```python
from build123d import *

# Parameters (mm, degrees)
F0_W      = 128
F0_H      = 175
F1_DEPTH  = 25
F2_T      = -2.5
F3_R      = 4
F3_R_2    = 1.5
F4_DEPTH  = 20
F7_DEPTH  = 25
F8_R      = 2
F9_DEPTH  = 25
F11_W     = 40
F11_H     = 74
F11_W_2   = 80
F11_H_2   = 15.985015
F12_DEPTH = 36
F13_R     = 1
F15_W     = 5.084744
F15_H     = 25.423729
F16_DEPTH = 47.5


with BuildPart() as f1:
    # F0 (on Front) → F1 (new body)
    with BuildSketch(Plane.XZ):
        Rectangle(F0_W, F0_H)
    extrude(amount=F1_DEPTH)

    # F2
    f2_openings = [f1.faces().sort_by_distance(p)[0] for p in [
        (0, -25, 0),
    ]]
    offset(amount=F2_T, openings=f2_openings)

    # F3 (on Front) → F4 (join)
    with BuildSketch(Plane.XZ):
        with Locations((-37, 47)):
            Circle(F3_R)
        with Locations((-37, 47)):
            Circle(F3_R_2, mode=Mode.SUBTRACT)
        with Locations((37, 47)):
            Circle(F3_R)
        with Locations((37, 47)):
            Circle(F3_R_2, mode=Mode.SUBTRACT)
        with Locations((37, -47)):
            Circle(F3_R)
        with Locations((37, -47)):
            Circle(F3_R_2, mode=Mode.SUBTRACT)
        with Locations((-37, -47)):
            Circle(F3_R)
        with Locations((-37, -47)):
            Circle(F3_R_2, mode=Mode.SUBTRACT)
    extrude(amount=F4_DEPTH)

    # F6 (on Front) → F7 (join)
    with BuildSketch(Plane.XZ):
        with BuildLine():
            Line((-61.93007, -75.520713), (-61.93007, -85.520713))
            Line((-61.93007, -85.520713), (-51.93007, -85.520713))
            ThreePointArc((-51.93007, -85.520713), (-54.690152, -78.280795), (-61.93007, -75.520713))
        make_face()
        with BuildLine():
            ThreePointArc((61.93007, -75.520713), (54.690152, -78.280795), (51.93007, -85.520713))
            Line((51.93007, -85.520713), (61.93007, -85.520713))
            Line((61.93007, -85.520713), (61.93007, -75.520713))
        make_face()
        with BuildLine():
            ThreePointArc((-61.6409, 75.150812), (-54.400982, 77.910894), (-51.6409, 85.150812))
            Line((-51.6409, 85.150812), (-61.6409, 85.150812))
            Line((-61.6409, 85.150812), (-61.6409, 75.150812))
        make_face()
        with BuildLine():
            Line((61.6409, 75.150812), (61.6409, 85.150812))
            Line((61.6409, 85.150812), (51.6409, 85.150812))
            ThreePointArc((51.6409, 85.150812), (54.400982, 77.910894), (61.6409, 75.150812))
        make_face()
    extrude(amount=F7_DEPTH)

    # F8 (on Front) → F9 (cut)
    with BuildSketch(Plane.XZ):
        with Locations((-58.5, 82)):
            Circle(F8_R)
        with Locations((-58.5, -82)):
            Circle(F8_R)
        with Locations((58.5, -82)):
            Circle(F8_R)
        with Locations((58.5, 82)):
            Circle(F8_R)
    extrude(amount=F9_DEPTH, mode=Mode.SUBTRACT)

    # F11 (on offset) → F12 (cut)
    with BuildSketch(Plane.XZ.offset(-10)):
        with Locations((-50, 0)):
            Rectangle(F11_W, F11_H)
        with Locations((50, 0)):
            Rectangle(F11_W, F11_H)
        with Locations((0, 67.007492)):
            Rectangle(F11_W_2, F11_H_2)
        with Locations((0, -67.007492)):
            Rectangle(F11_W_2, F11_H_2)
    extrude(amount=F12_DEPTH, mode=Mode.SUBTRACT)

    # F13
    f13_edges = [f1.edges().sort_by_distance(p)[0] for p in [
        (64, -12.5, 87.5),
        (0, 0, 87.5),
        (64, 0, 62.25),
        (64, 0, -62.25),
        (0, 0, -87.5),
        (-64, 0, 62.25),
        (-64, 0, -62.25),
        (-64, -12.5, 87.5),
    ]]
    fillet(f13_edges, radius=F13_R)

    # F15 (on Top) → F16 (cut)
    with BuildSketch(Plane.XY):
        with Locations((-63.120628, -15.211864)):
            Rectangle(F15_W, F15_H)
        with Locations((63.120628, -15.211864)):
            Rectangle(F15_W, F15_H)
    extrude(amount=-F16_DEPTH, mode=Mode.SUBTRACT)


solid = f1.part
```
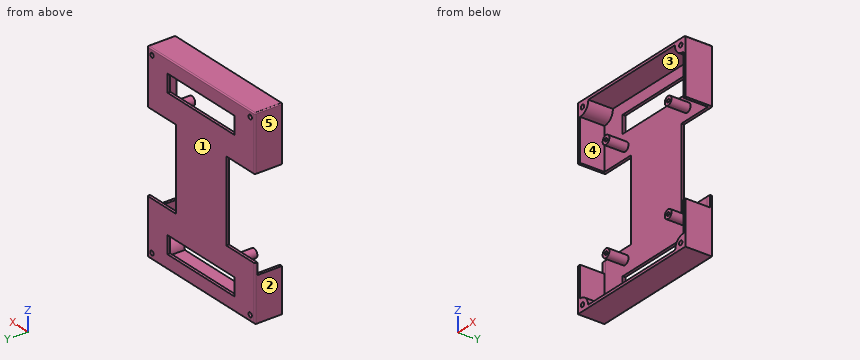
Input: part model. Units: mm. Frame: model coordinates. Face numbers are marked on the shaded views. A direction names the side the tool comes from. Round coordinates to 2 decimals unless told otherwise and drop trailing zeros. Loops run counter-clockwise (first coordinate to the right, second up) from the corner with the lowest first, then second, coordinate; pieces in that order, holes last. Notation, with made-up numbers: (67, 44.25) - (104, 44.25) arc R26 ccw to (104, 70.25) - close; hole circle Ø4 at (53.25, 37). An arc over 180 degrees is marked (long way). One line per item, written item: value. Start each with the question number.
(1) Draft query along X for the marked faces 1, 2 and 3. Return one class per face: +X half, -X half, draft (parallel to the pull), parting line (faces both ways), or undercut.
(2) Section B-B, the plane y = -23. Return loops of the section in (x, z).
(3) Access query for the marked faces 4 and 5. Directions: +Z, -Z, +X, -X, +Y, -Y. A direction counts if a zero-diameter tool reaches every point of the face in a straight line with its end or side. Return the directions, or none.
(4) Section D-D, the plane z = -82. Return loops of the section in (x, y).
(5) Section A-A, the plane y = -6.25. Count the separate pieces of the cut face and the enclosed holes in it, plus the area to 3 significant figures.
(6) Ray query, line 1 (Z direction, x = 37, y = -15.5); line 2 (X direction, y = -9.75, z = 47); line 3 (X direction, y = -15.5, z = -61.5). Return the intervals inside material, ascending. Write a range as [from, to].
(7) Contact query for flat-ended pins moving along their axis: P1, Ø3.5, axis at x = 58.5, z = -82, coming from the +Y side; P2, Ø2.5, axis at x = 39, z = -47, coming from the -Y side; P3, Ø1.7, axis at x = 62.5, z = -41.5, coming from the -Y side; P4, Ø0.8, axis at y = -0.5, z = -4, coming from the -X side. Output: stop coordinate, or through.
(8) Section C-C, the plane x = 2. Return loops of the section in (y, z), plus the area to 3 significant figures.
Results below:
1. face 1: draft
1. face 2: -X half
1. face 3: undercut
2. outline: (-64, -87.5) - (64, -87.5) - (64, -47.5) - (61.5, -47.5) - (61.5, -75.51) arc R9.48 ccw to (51.91, -85) - (-51.91, -85) arc R9.48 ccw to (-61.5, -75.51) - (-61.5, -47.5) - (-64, -47.5) - close; (-64, 37) - (-61.5, 37) - (-61.5, 75.14) arc R9.48 ccw to (-51.63, 85) - (51.63, 85) arc R9.48 ccw to (61.5, 75.14) - (61.5, 37) - (64, 37) - (64, 86.5) arc R1 ccw to (63, 87.5) - (-63, 87.5) arc R1 ccw to (-64, 86.5) - close; hole circle Ø4 at (-58.5, -82); hole circle Ø4 at (-58.5, 82); hole circle Ø4 at (58.5, -82); hole circle Ø4 at (58.5, 82)
3. face 4: -Y
3. face 5: +Z, -Z, -X, +Y, -Y
4. outline: (-64, -25) - (-60.5, -25) - (-60.5, 0) - (-63, 0) arc R1 ccw to (-64, -1) - close; (-56.5, -25) - (-52.4, -25) - (-52.4, -2.5) - (52.4, -2.5) - (52.4, -25) - (56.5, -25) - (56.5, 0) - (-56.5, 0) - close; (60.5, -25) - (64, -25) - (64, -1) arc R1 ccw to (63, 0) - (60.5, 0) - close
5. separate pieces: 6
5. enclosed holes: 8
5. area: 1,490 mm^2
6. line 1: [-87.5, -85], [-51, -48.5], [-45.5, -43], [43, 45.5], [48.5, 51], [85, 87.5]
6. line 2: [-64, -61.5], [-41, -38.5], [-35.5, -33], [33, 35.5], [38.5, 41], [61.5, 64]
6. line 3: [-64, -61.5], [61.5, 64]
7. P1: through
7. P2: y = -20
7. P3: y = -2.5
7. P4: x = -30
8. outline: (-25, -87.5) - (-1, -87.5) arc R1 ccw to (0, -86.5) - (0, -75) - (-2.5, -75) - (-2.5, -85) - (-25, -85) - close; (-25, 85) - (-2.5, 85) - (-2.5, 75) - (0, 75) - (0, 86.5) arc R1 ccw to (-1, 87.5) - (-25, 87.5) - close; (-2.5, -59.01) - (0, -59.01) - (0, 59.01) - (-2.5, 59.01) - close
8. area: 470 mm^2
